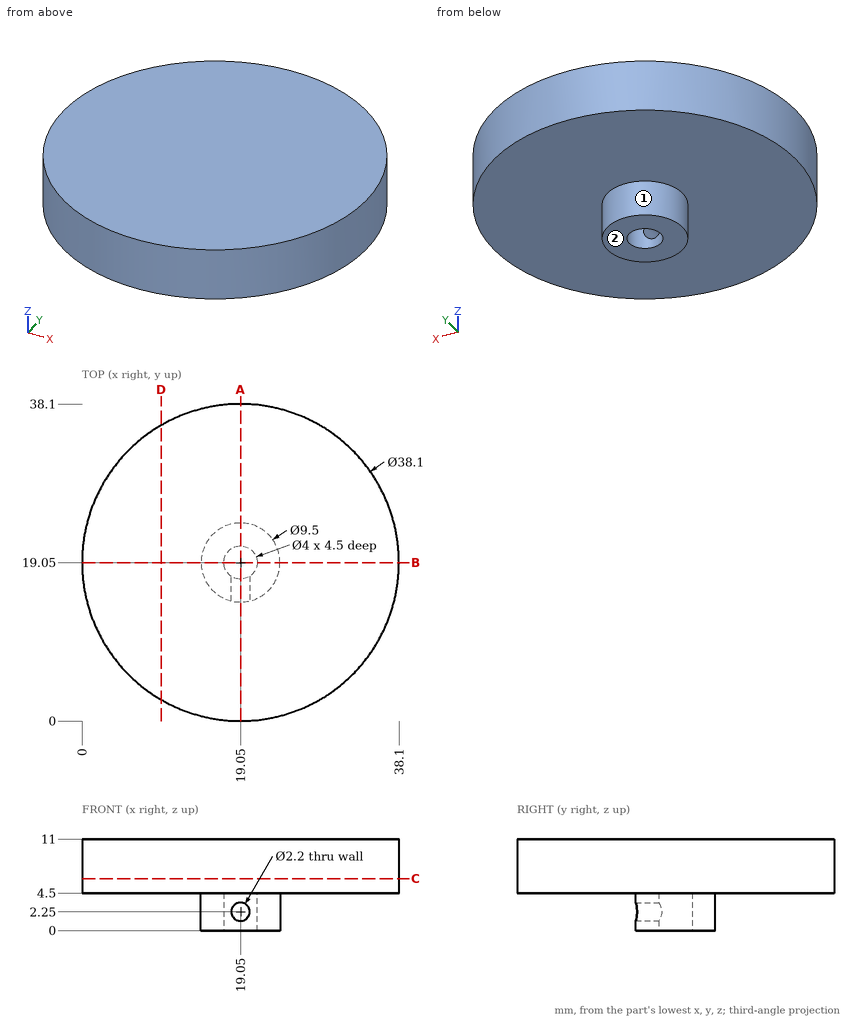
Geometry: see drawing. Coordinates: mm, zero at the bounding-box minimum. A direction names the side the tool comes from. Give positions to 0.01 mm unless a question says otherwise; leave off trailing zeros. Write each loop counter-clockwise with the first axis right and the second up, starting at its lowest first coordinate (ties: lowest second). Pieces come first, ordered by that corner, then holes. Notation, with made-up numbers: M 24,31 L 64,31 A21 ccw 64,50 Z; hole C -16.5,-4 d9. An arc over 180 degrees is marked long. Answer in a Markdown table with one row per item. Add a question column.
(1) First-contact query: pin 1 (1 mm diameter, centred on x = 21.5, z = 2.5, fed in from -Y); pin 2 (1 mm diameter, centred on y = 30.5, z = 4.5, fed in from +X); pin 3 (6 mm diameter, centred on y = 20, z = 4.5, fed in from -X); pin 4 (3 mm diameter, centred on x = 19.05, z = 2.25, fed in from -Y). Flat tips, straight axial feed; report the tip coordinate or a pass-through.
(2) Section C-C on z = 6.25. Return loops of the section in (x, y), and give its area (3 significant figures).
(3) Section D-D on x = 9.5. Return loops of the section in (y, z).
(4) Section B-B on y = 19.05. Return loops of the section in (x, z).
(5) Reachability of the marked faces 1 and 2 from +Z, -Z, +X, -X, +Y, -Y: full face, straight path, thin tool, end or side. Return the list, or none.
(6) Section A-A on x = 19.05. Return loops of the section in (y, z).
(7) Ray query, line 1 (Z direction, x = 19.05, y = 16.3); line 2 (Y direction, x = 19.05, z = 3.55); line 3 (Z direction, x = 31.5, y = 24). Return the intervals inside material, ascending.
Result set:
| question | item | result |
|---|---|---|
| 1 | pin 1 | stops at y = 14.72 |
| 1 | pin 2 | stops at x = 34.64 |
| 1 | pin 3 | stops at x = 0 |
| 1 | pin 4 | stops at y = 14.3 |
| 2 | outline | C 19.05,19.05 d38.1 |
| 2 | area | 1,140 mm^2 |
| 3 | outline | M 2.57,4.5 L 35.53,4.5 L 35.53,11 L 2.57,11 Z |
| 4 | outline | M 0,4.5 L 14.3,4.5 L 14.3,0 L 17.05,0 L 17.05,4.5 L 21.05,4.5 L 21.05,0 L 23.8,0 L 23.8,4.5 L 38.1,4.5 L 38.1,11 L 0,11 Z |
| 5 | face 1 | -Z |
| 5 | face 2 | -Z, +X, -X, +Y, -Y |
| 6 | outline | M 0,4.5 L 14.3,4.5 L 14.3,3.35 L 17.05,3.35 L 17.05,4.5 L 21.05,4.5 L 21.05,0 L 23.8,0 L 23.8,4.5 L 38.1,4.5 L 38.1,11 L 0,11 Z; M 14.3,0 L 17.05,0 L 17.05,1.15 L 14.3,1.15 Z |
| 7 | line 1 | z = 0 to 1.15, 3.35 to 11 |
| 7 | line 2 | y = 14.3 to 17.05, 21.05 to 23.8 |
| 7 | line 3 | z = 4.5 to 11 |
